Source: CAD feature listing. Evaluate the final solid. Frame: model axes, mm. A direction names the side the tool comes from. Coordinates: 2 decimals unless noted, no trailing zeros. Order: outer loops, then holes, each group sorted by start corner. A loop starts at its lowest first (then second) coordinate and runs counter-clockwise, first axis right, second up. Notation, with made-up numbers: (36, 34) -> (64, 34) arc R22 cw to (64, 41) -> close; hole circle Ø9 at (-31.5, 64). An arc over 180 degrees is marked (long way). Put each result on its own line as item: value.
from build123d import *

# Parameters (mm, degrees)
SKETCH_1_W          = 55
SKETCH_1_H          = 75
EXTRUDE_1_DEPTH     = 1
SKETCH_3_W          = 48
SKETCH_3_H          = 65
SKETCH_3_W_2        = 46
SKETCH_3_H_2        = 63
EXTRUDE_2_DEPTH     = 5
SKETCH_4_W          = 7
SKETCH_4_H          = 2.5
EXTRUDE_3_DEPTH     = 3
SKETCH_5_R          = 1.9
EXTRUDE_4_DEPTH     = 23
SKETCH_6_R          = 0.75
CUT_EXTRUDE_1_DEPTH = 10
SKETCH_7_R          = 2
EXTRUDE_5_DEPTH     = 23
SKETCH_8_R          = 0.75
CUT_EXTRUDE_2_DEPTH = 10
CHAMFER_1_SIZE      = 1.5
FILLET_2_R          = 1


with BuildPart() as part:
    # Эскиз1 → Бобышка-Вытянуть1 (new body)
    with BuildSketch(Plane(origin=(0, 0, 0), x_dir=(1, 0, 0), z_dir=(0, 1, 0))):
        with Locations((0.630718954, -16.009803922)):
            Rectangle(SKETCH_1_W, SKETCH_1_H)
    extrude(amount=-EXTRUDE_1_DEPTH)

    # Эскиз3 → Бобышка-Вытянуть2 (add)
    with BuildSketch(Plane(origin=(0, 0, 0), x_dir=(1, 0, 0), z_dir=(0, 1, 0))):
        with Locations((1.423879909, -15.093947699)):
            Rectangle(SKETCH_3_W, SKETCH_3_H)
        with Locations((1.423879909, -15.093947699)):
            Rectangle(SKETCH_3_W_2, SKETCH_3_H_2, mode=Mode.SUBTRACT)
    extrude(amount=EXTRUDE_2_DEPTH)

    # Эскиз4 → Бобышка-Вытянуть3 (add)
    with BuildSketch(Plane(origin=(0, 0, 0), x_dir=(1, 0, 0), z_dir=(0, 1, 0))):
        with Locations((1.423879909, -45.343947699)):
            Rectangle(SKETCH_4_W, SKETCH_4_H)
        with Locations((0.74590962, 15.156052301)):
            Rectangle(SKETCH_4_W, SKETCH_4_H)
    extrude(amount=EXTRUDE_3_DEPTH)

    # Эскиз5 → Бобышка-Вытянуть4 (add)
    with BuildSketch(Plane(origin=(0, 0, 0), x_dir=(1, 0, 0), z_dir=(0, 1, 0))):
        with Locations((1.423879909, -39.643947699)):
            Circle(SKETCH_5_R)
    extrude(amount=EXTRUDE_4_DEPTH)

    # Эскиз6 → Вырез-Вытянуть1 (cut)
    with BuildSketch(Plane(origin=(0, 23, 0), x_dir=(1, 0, 0), z_dir=(0, 1, 0))):
        with Locations((1.423879909, -39.643947699)):
            Circle(SKETCH_6_R)
    extrude(amount=-CUT_EXTRUDE_1_DEPTH, mode=Mode.SUBTRACT)

    # Эскиз7 → Бобышка-Вытянуть5 (add)
    with BuildSketch(Plane(origin=(0, 0, 0), x_dir=(1, 0, 0), z_dir=(0, 1, 0))):
        with Locations((1.423879909, 8.406052301)):
            Circle(SKETCH_7_R)
    extrude(amount=EXTRUDE_5_DEPTH)

    # Эскиз8 → Вырез-Вытянуть2 (cut)
    with BuildSketch(Plane(origin=(0, 23, 0), x_dir=(1, 0, 0), z_dir=(0, 1, 0))):
        with Locations((1.423879909, 8.406052301)):
            Circle(SKETCH_8_R)
    extrude(amount=-CUT_EXTRUDE_2_DEPTH, mode=Mode.SUBTRACT)

    # Фаска1
    chamfer_1_edges = [part.edges().sort_by_distance(p)[0] for p in [
        (-22.576120091, 0, 15.093947699),
        (1.423879909, 0, 47.593947699),
        (25.423879909, 0, 15.093947699),
        (1.423879909, 0, -17.406052301),
    ]]
    chamfer(chamfer_1_edges, length=CHAMFER_1_SIZE)

    # Скругление2
    fillet_2_edges = [part.edges().sort_by_distance(p)[0] for p in [
        (-23.326120091, 0.75, -18.156052301),
        (26.173879909, 0.75, -18.156052301),
        (-23.326120091, 0.75, 48.343947699),
        (26.173879909, 0.75, 48.343947699),
    ]]
    fillet(fillet_2_edges, radius=FILLET_2_R)


solid = part.part
1. Set-up query: faces 1 (the flat face through (-2.076, 1, 45)), 2 (the flat face through (1.4, 23, -7.5)). Return all of +Z, -Z, +X, -X, +Y, -Y with unobstructed straight access to the full face (end or side cutting, diameter ignored); none if empty.
Numbers:
face 1: +Y
face 2: +Z, -Z, +X, -X, +Y
2. Ray query, line 1 along Z through (x, y) = (-11, 4.5); line 2 along Y through (x, z) = (-7, 29); line 3 along Y through (x, z) = (20, 47.5). Return the intervals inside material, ascending.
Numbers:
line 1: z = -17.41 to -16.41, 46.59 to 47.59
line 2: y = -1 to 0
line 3: y = -1 to 5
3. Cut plane C-C on y = 16.5. Output: boundary loops of the cut face in (x, z).
Numbers:
outline: circle Ø4 at (1.42, -8.41); circle Ø3.8 at (1.42, 39.64); hole circle Ø1.5 at (1.42, -8.41); hole circle Ø1.5 at (1.42, 39.64)
4. Cut plane B-B on x = 20. Output: boundary loops of the cut face in (y, z).
Numbers:
outline: (-1, -21.49) -> (0, -21.49) -> (0, -18.91) -> (1.5, -17.41) -> (5, -17.41) -> (5, -16.41) -> (0, -16.41) -> (0, 46.59) -> (5, 46.59) -> (5, 47.59) -> (1.5, 47.59) -> (0, 49.09) -> (0, 53.51) -> (-1, 53.51) -> close
5. Pull-direction query (Z, two-part tool) for faces 3 (the flat face through (-22.576, 4, 16)), 4 (the flat face through (1, 3, 47.594)), 5 (the flat face through (24.424, 2, 16)); classes: pulls with the +Z half, pulls with the -Z half, needs draft (parallel to the pull), parting line crosses it, or undercut.
Numbers:
face 3: needs draft
face 4: pulls with the +Z half
face 5: undercut
6. Cut plane D-D on y = 6.5. Output: boundary loops of the cut face in (x, z).
Numbers:
outline: circle Ø4 at (1.42, -8.41); circle Ø3.8 at (1.42, 39.64)
7. Cut plane A-A on z = 4.5. Output: boundary loops of the cut face in (x, y), plus the area to 4 significant figures.
Numbers:
outline: (-26.87, -1) -> (28.13, -1) -> (28.13, 0) -> (26.92, 0) -> (25.42, 1.5) -> (25.42, 5) -> (24.42, 5) -> (24.42, 0) -> (-21.58, 0) -> (-21.58, 5) -> (-22.58, 5) -> (-22.58, 1.5) -> (-24.08, 0) -> (-26.87, 0) -> close
area: 67.25 mm2
8. First-contact query: pin 1 (1.8 mm diameter, centred on x = -4, y = 4, fed in from -Z); pin 2 (5 mm diameter, centred on y = 3, z = 11.5, fed in from -X); pin 3 (10 mm diameter, centred on y = 16, z = 29, fed in from +X); pin 4 (1.5 mm diameter, centred on y = 2, z = 8, fed in from +X). Flat tips, straight axial feed; report the tip coordinate or a pass-through.
Numbers:
pin 1: stops at z = -17.41
pin 2: stops at x = -23.58
pin 3: passes through
pin 4: stops at x = 25.67
